```python
from build123d import *

# Parameters (mm, degrees)
BOSS_EXTRUDE1_DEPTH = 1.524


with BuildPart() as part:
    # Sketch1 → Boss-Extrude1 (new body)
    with BuildSketch(Plane.XY):
        with BuildLine():
            Line((-12.390496283, 0), (-12.390496283, -1.524))
            Line((-12.390496283, -1.524), (-11.440495099, -1.524))
            ThreePointArc((-11.440495099, -1.524), (-13.160567298, -3.340075702), (-15.652172906, -3.560713016))
            ThreePointArc((-15.652172906, -3.560713016), (-16.43578107, -1.039818757), (-17.898233983, 1.157948542))
            ThreePointArc((-17.898233983, 1.157948542), (-34.014860834, 24.840522989), (-41.571298491, 52.472212106))
            ThreePointArc((-41.571298491, 52.472212106), (-41.120011165, 54.045320934), (-39.952895072, 55.192566182))
            ThreePointArc((-39.952895072, 55.192566182), (-40.500139361, 53.88401522), (-40.636498822, 52.472212106))
            ThreePointArc((-40.636498822, 52.472212106), (-32.67469804, 25.640883384), (-15.652172906, 3.425030694))
            ThreePointArc((-15.652172906, 3.425030694), (-15.109824899, 2.798358256), (-14.338010517, 2.496427364))
            ThreePointArc((-14.338010517, 2.496427364), (-12.609091081, 1.573387542), (-11.440495099, 0))
            Line((-11.440495099, 0), (-12.390496283, 0))
        make_face()
    extrude(amount=BOSS_EXTRUDE1_DEPTH)


solid = part.part
```
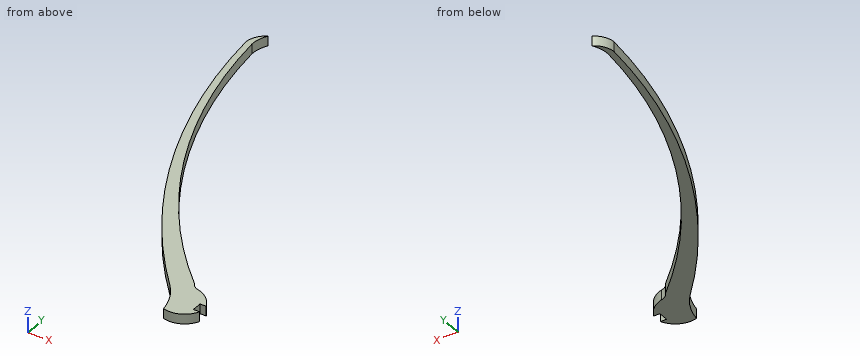
Geometry check sheet. Reference: the model listing, model coordinates, mm. Round coordinates to 2 decimals unless told otherwise and drop trailing zeros. Order: outer loops, then holes, each group sorted by start corner. A loop starts at its lowest first (then second) coordinate and runs counter-clockwise, first axis right, second up. Notation, with made-up numbers: (-20, -6) -> (5, -6) arc R30 cw to (5, 20) -> close; hole circle Ø9 at (-22.5, 15.25). An arc over 180 degrees is marked (long way). Return JSON: item names as keys, results as strings. Group by question number.
Q1. Section check B-B, the plane y = 36.5. Record the boundary of the cut face in (x, z), plus the area to 3 significant figures.
Q2. Gauge pin test, flat end, axial feed: pin 1 (0.8 mm diameter, centred on x = -11.5, z = 0.5, fed in from +Y). Record the tip position at first contact, or that the pin passes through.
Q3. Material ranges on probe 1 along X at (y, z) = (31, 1.1); probe 2 along X at (y, z) = (51, 0.1); probe 3 along Y at (x, z) = (-35.5, 1.2), recorded low to high. Write a range as from..to.
Q4. Section check A-A, the plane z = 0.25. Record the boundary of the cut face in (x, y) (1 decimal).
Q5. Section check C-C, the plane x = -36. Record the boundary of the cut face in (y, z), plus the area to 3 significant figures.
Numbers:
{
 "1": {"outline": "(-38.41, 0) -> (-37.2, 0) -> (-37.2, 1.52) -> (-38.41, 1.52) -> close", "area": "1.85 mm^2"},
 "2": {"pin 1": "y = 0.8"},
 "3": {"probe 1": "-36.57..-35.15", "probe 2": "-41.41..-40.47", "probe 3": "28.25..31.85"},
 "4": {"outline": "(-41.6, 52.5) arc R87 ccw to (-17.9, 1.2) arc R9.3 cw to (-15.7, -3.6) arc R3.5 ccw to (-11.4, -1.5) -> (-12.4, -1.5) -> (-12.4, 0) -> (-11.4, 0) arc R4.5 ccw to (-14.3, 2.5) arc R1.7 cw to (-15.7, 3.4) arc R77 cw to (-40.6, 52.5) arc R4.7 cw to (-40, 55.2) arc R3.2 ccw to start"},
 "5": {"outline": "(29.49, 0) -> (33.13, 0) -> (33.13, 1.52) -> (29.49, 1.52) -> close", "area": "5.54 mm^2"}
}
